Autodesk Inventor part; units mm, degrees
ref_plane "YZ Plane" through (0, 0, 0) normal (1, 0, 0) x (0, 1, 0)
ref_plane "XZ Plane" through (0, 0, 0) normal (0, 1, 0) x (-1, 0, 0)
ref_plane "XY Plane" through (0, 0, 0) normal (0, 0, 1) x (1, 0, 0)
sketch "Sketch1" plane through (0, 0, 0) normal (0, 1, 0) x (-1, 0, 0)
  line L0 (0, 0) -> (0, -261.6) construction
  line L1 (5, 0) -> (5, -261.6)
  line L2 (-5, -261.6) -> (-5, 0)
  arc A0 (5, 0) -> (-5, 0) centre (0, 0) ccw
  arc A1 (-5, -261.6) -> (5, -261.6) centre (0, -261.6) ccw
  circle A2 centre (0, 0) radius 1.65
  circle A3 centre (0, -261.6) radius 1.65
  circle A4 centre (0, -153.559) radius 1.65
  point P0 (0, -130.8)
  dimension "d0" = 3.3
  dimension "d1" = 3.3
  dimension "d2" = 10
  dimension "d3" = 261.6
  dimension "d4" = 3.3
  dimension "d5" = 153.559
extrude "Extrusion1" add sketch "Sketch1" along normal blind 3
sketch "Sketch3" plane through (0, 3, 0) normal (0, 1, 0) x (1, 0, 0)
  line L0 (-22.4574, 275.926) -> (26.2563, 275.926)
  line L1 (26.2563, 275.926) -> (26.2563, 121.3008)
  line L2 (26.2563, 121.3008) -> (-22.4574, 121.3008)
  line L3 (-22.4574, 121.3008) -> (-22.4574, 275.926)
  line L4 (-103.4002, 357.0257) -> (155.5228, 357.0257)
  line L5 (155.5228, 357.0257) -> (155.5228, -67.8162)
  line L6 (155.5228, -67.8162) -> (-103.4002, -67.8162)
  line L7 (-103.4002, -67.8162) -> (-103.4002, 357.0257)
  point P0 (0, 0)
extrude "Extrusion2" cut sketch "Sketch3" against normal blind 100 contours L0 L1 L2 L3
properties part number "Part_2_p1"
CAD build for the part. Positions are in the model's coordinates, mm. Round coordinates to 2 decimals unless told otherwise and drop trailing zeros. Order: outer loops, then holes, each group sorted by start corner. A loop starts at its lowest first (then second) coordinate and runs counter-clockwise, first axis right, second up.
Q1. Slice it at A-A (x = 0). Write the cut outline in (y, z).
Q2. Two-plate mould, pull along X, no slides. Class faces 1 (the flat face through (0, 3, -57)), 2 (the flat face through (5, 1, -61)), 3 (the cylindrical face through (1.216, 1.479, -1.115)), 4 (the flat face through (-5, 1, -60)): pulls with the +X half, pulls with the -X half, needs draft (parallel to the pull), parting line crosses it, or undercut.
Q3. Drop a flat-ended pin along its axis: pin 1 (1.5 mm diameter, centred on x = 3, y = 2.5, fed in from +Z). Give the stop position or say it passes through.
Q4. Wall check: L1, parallel to Z at x = -0.25, y = 2.75; L2, parallel to Z at x = -0.75, y = 2.15; L3, parallel to Z at x = 3.25, y = 0.2. Give the ranges that are in metal, low to high.
Q5. Slice it at B-B (y = 0.65). Write the cut outline in (x, z), and give its area (3 significant figures).
Results below:
1. outline: (0, -121.3) - (3, -121.3) - (3, -1.65) - (0, -1.65) - close; (0, 1.65) - (3, 1.65) - (3, 5) - (0, 5) - close
2. face 1: needs draft
2. face 2: pulls with the +X half
2. face 3: undercut
2. face 4: pulls with the -X half
3. pin 1: stops at z = 4.47
4. L1: z = -121.3 to -1.63, 1.63 to 4.99
4. L2: z = -121.3 to -1.47, 1.47 to 4.94
4. L3: z = -121.3 to 3.8
5. outline: (-5, -121.3) - (5, -121.3) - (5, 0) arc R5 ccw to (-5, 0) - close; hole circle Ø3.3 at (0, 0)
5. area: 1,240 mm2
